Read the model definition and answer for the solid it produces. Units are mm, in the model's axes. Give positions to 0.01 mm unless a question says otherwise; leave off trailing zeros. Order: outer loops, then holes, each group sorted by start corner. A loop starts at its lowest first (then second) coordinate and runs counter-clockwise, first axis right, second up. Notation, with made-up numbers: (3.5, 9) -> (25.5, 9) arc R18 ccw to (25.5, 29) -> close; hole circle Ø2 at (44.25, 60.5). An arc over 180 degrees is marked (long way). One line per question, with ' | ' between items. Start each with the question number.
Autodesk Inventor part; units mm, degrees
ref_plane "YZ Plane" through (0, 0, 0) normal (1, 0, 0) x (0, 1, 0)
ref_plane "XZ Plane" through (0, 0, 0) normal (0, 1, 0) x (-1, 0, 0)
ref_plane "XY Plane" through (0, 0, 0) normal (0, 0, 1) x (1, 0, 0)
sketch "スケッチ1" plane through (0, 0, 0) normal (0, 0, 1) x (1, 0, 0)
  line L0 (18, 0) -> (18, 100)
  line L1 (0, 100) -> (0, 0)
  line L2 (9, 100) -> (9, 0) construction
  arc A0 (18, 100) -> (0, 100) centre (9, 100) ccw
  arc A1 (0, 0) -> (18, 0) centre (9, 0) ccw
  circle A2 centre (9, 0) radius 3.5
  circle A3 centre (9, 100) radius 3.5
  circle A4 centre (9, 50) radius 3.5
  dimension "d35" = 18
  dimension "d36" = 100
  dimension "d37" = 7
  dimension "d38" = 7
  dimension "d41" = 7
extrude "押し出し1" add sketch "スケッチ1" along normal blind 2
properties part number "hip_link" material "GFRP"
Q1. A cutting plane is placed at C-C, the plane z = 0.85. Determine the outline of the cut face in (x, y), then the cut area to 3 significant figures.
Q2. A cutting plane is placed at D-D, the plane y = 1. Determine the outline of the cut face in (x, z), then the cut area to 3 significant figures.
Q3. Determine the mould class of faces 1 (the cylindrical face through (9, -9, 1)), 2 (the flat face through (18, 49, 1)), 3 (the cylindrical face through (8.54, 46.53, 0.99)), 4 (the cylindrical face through (8.241, 103.417, 0.986)) for opening direction Y: pulls with the +Y half, pulls with the -Y half, needs draft (parallel to the pull), parting line crosses it, or undercut.
Q4. A cutting plane is placed at A-A, the plane x = 9. Determine the outline of the cut face in (y, z).
Q5. A cutting plane is placed at B-B, the plane y = 50. Determine the outline of the cut face in (x, z).
Q6. Find the intervals of material crossed by line 1 (Y direction, x = 9, z = 1.15); line 2 (Y direction, x = 8, z = 0.9); line 3 (X direction, y = 98, z = 1.2), in increasing order.
Geometry results:
1) outline: (0, 0) arc R9 ccw to (18, 0) -> (18, 100) arc R9 ccw to (0, 100) -> close; hole circle Ø7 at (9, 0); hole circle Ø7 at (9, 50); hole circle Ø7 at (9, 100) | area: 1,940 mm²
2) outline: (0, 0) -> (5.65, 0) -> (5.65, 2) -> (0, 2) -> close; (12.35, 0) -> (18, 0) -> (18, 2) -> (12.35, 2) -> close | area: 22.6 mm²
3) face 1: pulls with the -Y half | face 2: needs draft | face 3: undercut | face 4: undercut
4) outline: (-9, 0) -> (-3.5, 0) -> (-3.5, 2) -> (-9, 2) -> close; (3.5, 0) -> (46.5, 0) -> (46.5, 2) -> (3.5, 2) -> close; (53.5, 0) -> (96.5, 0) -> (96.5, 2) -> (53.5, 2) -> close; (103.5, 0) -> (109, 0) -> (109, 2) -> (103.5, 2) -> close
5) outline: (0, 0) -> (5.5, 0) -> (5.5, 2) -> (0, 2) -> close; (12.5, 0) -> (18, 0) -> (18, 2) -> (12.5, 2) -> close
6) line 1: -9 to -3.5, 3.5 to 46.5, 53.5 to 96.5, 103.5 to 109 | line 2: -8.94 to -3.35, 3.35 to 46.65, 53.35 to 96.65, 103.35 to 108.94 | line 3: 0 to 6.13, 11.87 to 18
